Could you check a few things on this drawing? It's one solid part, dimensions in mm from its lowest x, y, z. A direction names the side the tool comes from. Round coordinates to 2 decimals unless told otherwise and drop trailing zeros. Loops run counter-clockwise (first coordinate to the right, second up) from the corner with the lowest first, then second, coordinate; pieces in that order, holes last.
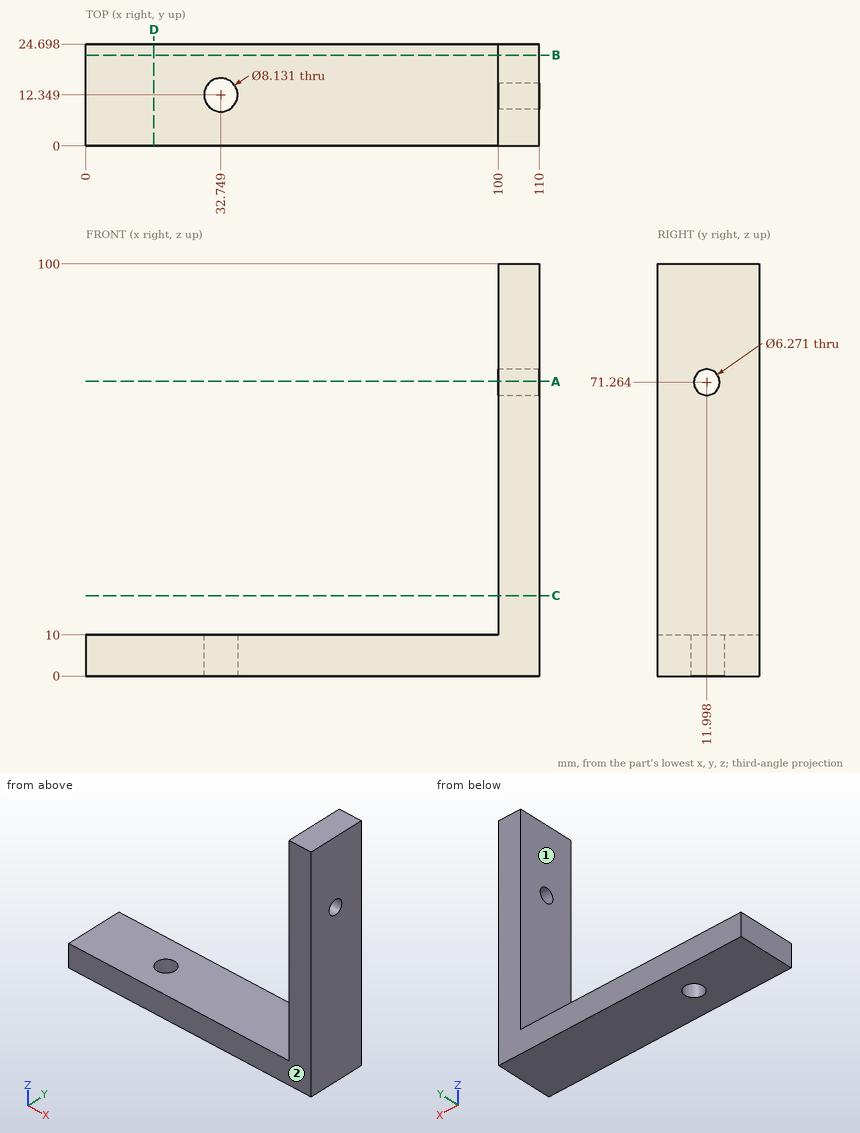
(1) Suppose I cut it at A-A (z = 71.5). Write out the boundary of the cut face in (x, y) (1 decimal).
(2) Which directions (+Z, -Z, +X, -X, +Y, -Y) give clear straight access to the entire face, cutting with the end or side of a thin tool? Please do the marked faces 1 and 2.
(3) If I drill on line 1 (Z direction, x = 97, y = 15.5); line 2 (X direction, y = 5, z = 66), over which ranges is the centre line in solid material (lowest first)?
(4) Suppose I cut it at D-D (x = 16.5). Write out the boundary of the cut face in (y, z).
(5) Suppose I cut it at B-B (y = 22). Write out the boundary of the cut face in (x, z).
(6) Suppose I cut it at C-C (z = 19.5). Write out the boundary of the cut face in (x, y).
(7) For pin 1 (10 mm diameter, centred on y = 11.5, z = 40.5, fed in from -X); pin 2 (12.5 mm diameter, centred on x = 48.5, y = 11.5, fed in from +Z), each with a flat end and sliding along its axis, tell me the tip position at first contact or that it passes through.
Check result:
1. outline: (100, 0) - (110, 0) - (110, 8.9) - (100, 8.9) - close; (100, 15.1) - (110, 15.1) - (110, 24.7) - (100, 24.7) - close
2. face 1: +Z, -X, +Y, -Y
2. face 2: +Z, -Z, +X, -X, -Y
3. line 1: z = 0 to 10
3. line 2: x = 100 to 110
4. outline: (0, 0) - (24.7, 0) - (24.7, 10) - (0, 10) - close
5. outline: (0, 0) - (110, 0) - (110, 100) - (100, 100) - (100, 10) - (0, 10) - close
6. outline: (100, 0) - (110, 0) - (110, 24.7) - (100, 24.7) - close
7. pin 1: stops at x = 100
7. pin 2: stops at z = 10
